from build123d import *

# Parameters (mm, degrees)
EXTRUDE_1_DEPTH     = 20
SKETCH_2_R          = 7
CUT_EXTRUDE_1_DEPTH = 21
SKETCH_3_W          = 30
SKETCH_3_H          = 8
CUT_EXTRUDE_2_DEPTH = 21
FILLET_1_R          = 4
CHAMFER_1_SIZE      = 0.5
M4X0_71_D           = 3.3
M4X0_71_DEPTH       = 13.5
M4X0_71_TIP         = 0.991420021
SKETCH_6_R          = 2
CUT_EXTRUDE_3_DEPTH = 5
SKETCH_7_R          = 2
CUT_EXTRUDE_4_DEPTH = 5
SKETCH_8_R          = 2
EXTRUDE_2_DEPTH     = 5
SKETCH_9_R          = 2
EXTRUDE_3_DEPTH     = 5


with BuildPart() as part:
    # Эскиз1 → Бобышка-Вытянуть1 (new body)
    with BuildSketch(Plane(origin=(0, 0, 0), x_dir=(1, 0, 0), z_dir=(0, 1, 0))):
        with BuildLine():
            Line((0, 0), (14.43375673, -25))
            Line((14.43375673, -25), (65.56624327, -25))
            Line((65.56624327, -25), (80, 0))
            Line((80, 0), (73.07179677, 4))
            Line((73.07179677, 4), (63.396104176, -12.758791171))
            ThreePointArc((63.396104176, -12.758791171), (56.617091212, -7.146468727), (48.291796068, -10))
            Line((48.291796068, -10), (31.708203932, -10))
            ThreePointArc((31.708203932, -10), (23.382908788, -7.146468727), (16.603895824, -12.758791171))
            Line((16.603895824, -12.758791171), (6.92820323, 4))
            Line((6.92820323, 4), (0, 0))
        make_face()
    extrude(amount=EXTRUDE_1_DEPTH)

    # Эскиз2 → Вырез-Вытянуть1 (cut, through all)
    with BuildSketch(Plane(origin=(0, 20, 0), x_dir=(1, 0, 0), z_dir=(0, 1, 0))):
        with Locations((25, -16)):
            Circle(SKETCH_2_R)
        with Locations((55, -16)):
            Circle(SKETCH_2_R)
    extrude(amount=-CUT_EXTRUDE_1_DEPTH, mode=Mode.SUBTRACT)

    # Эскиз3 → Вырез-Вытянуть2 (cut, through all)
    with BuildSketch(Plane(origin=(0, 20, 0), x_dir=(1, 0, 0), z_dir=(0, 1, 0))):
        with Locations((40, -16)):
            Rectangle(SKETCH_3_W, SKETCH_3_H)
    extrude(amount=-CUT_EXTRUDE_2_DEPTH, mode=Mode.SUBTRACT)

    # Скругление1
    fillet_1_edges = [part.edges().sort_by_distance(p)[0] for p in [
        (6.92820323, 10, -4),
        (16.603895824, 10, 12.758791171),
        (31.708203932, 10, 10),
        (48.291796068, 10, 10),
        (63.396104176, 10, 12.758791171),
        (73.07179677, 10, -4),
        (65.56624327, 10, 25),
        (14.43375673, 10, 25),
        (49.255437353, 10, 12),
        (49.255437353, 10, 20),
        (30.744562647, 10, 20),
        (30.744562647, 10, 12),
    ]]
    fillet(fillet_1_edges, radius=FILLET_1_R)

    # Фаска1
    chamfer_1_edges = [part.edges().sort_by_distance(p)[0] for p in [
        (80, 10, 0),
        (0, 10, 0),
    ]]
    chamfer(chamfer_1_edges, length=CHAMFER_1_SIZE)

    # Отверстие обработанное метчиком M4x0.71
    with Locations(Plane(origin=(40, 5, 10), x_dir=(-1, 0, 0), z_dir=(0, 0, -1))):
        with Locations((0, 0), (0, 10)):
            Hole(M4X0_71_D / 2, depth=M4X0_71_DEPTH)
            with Locations((0, 0, -(M4X0_71_DEPTH + M4X0_71_TIP / 2))):  # 118° drill point
                Cone(0, M4X0_71_D / 2, M4X0_71_TIP, mode=Mode.SUBTRACT)

    # Эскиз6 → Вырез-Вытянуть3 (cut)
    with BuildSketch(Plane(origin=(60, 0, 34.641016151), x_dir=(0.5, 0, -0.866025404), z_dir=(0.866025404, 0, 0.5))):
        with Locations((23.441887617, 10)):
            Circle(SKETCH_6_R)
    extrude(amount=-CUT_EXTRUDE_3_DEPTH, mode=Mode.SUBTRACT)

    # Эскиз7 → Вырез-Вытянуть4 (cut)
    with BuildSketch(Plane(origin=(0, 0, 0), x_dir=(0.5, 0, 0.866025404), z_dir=(-0.866025404, 0, 0.5))):
        with Locations((16.558112383, 10)):
            Circle(SKETCH_7_R)
    extrude(amount=-CUT_EXTRUDE_4_DEPTH, mode=Mode.SUBTRACT)

    # Эскиз8 → Бобышка-Вытянуть2 (add)
    with BuildSketch(Plane(origin=(0, 0, 0), x_dir=(0.5, 0, 0.866025404), z_dir=(-0.866025404, 0, 0.5))):
        with Locations((5, 16)):
            Circle(SKETCH_8_R)
    extrude(amount=EXTRUDE_2_DEPTH)

    # Эскиз9 → Бобышка-Вытянуть3 (add)
    with BuildSketch(Plane(origin=(60, 0, 34.641016151), x_dir=(0.5, 0, -0.866025404), z_dir=(0.866025404, 0, 0.5))):
        with Locations((35, 16)):
            Circle(SKETCH_9_R)
    extrude(amount=EXTRUDE_3_DEPTH)


solid = part.part
Verification items for the finished model (mm, model axes). A direction names the side the tool comes from. Give positions to 0.01 mm unless a question says otherwise; leave off trailing zeros. Order: outer loops, then holes, each group sorted by start corner. A loop starts at its lowest first (then second) coordinate and runs counter-clockwise, first axis right, second up. Notation, with made-up numbers: M -5,61.25 L 46,61.25 A17 cw 46,89.25 Z; hole C 40,76.5 d5. An arc over 180 degrees is marked long. Answer as a JSON object with one key per item and string values. Group by question number.
1) Cross-section at A-A (x = 55). Enter the section's corners in (y, z).
2) Cross-section at B-B (x = 26.5). Enter the section's corners in (y, z).
3) Access from +Z, -Z, +X, -X, +Y, -Y to the whole of each face (thin tool, end or side, straight path). Record for faces 4 (the face through (40, 10, 25)), 5 (the face through (38.35, 5.07, 21.77)), 6 (the face through (67.38, 10.03, 11.86)), 7 (the face through (62, 10, 16)), 8 (the face through (40, 10, 10)).
4) Depth check by flat-ended pin: pin 1 Ø6 at (x, y) = (73, 11.5) entering from +Z; pin 2 Ø3 at (y, z) = (17.5, 6.5) entering from +X; pin 3 Ø2.5 at (x, y) = (40, 5) entering from -Z; pin 4 Ø8.5 at (x, z) = (55, 16) entering from +Y. Enter the tip coordinate at first touch or a pass-through.
5) Scan lines: line 1 along Y through (x, z) = (40, 10.6); line 2 along Z through (x, y) = (54.5, 3.5); line 3 along X through (y, z) = (17.75, 7.75). Record each from-to range of solid material in increasing order. Write a range as [from, to].
6) Mould release check, pull along Z, two halves, no side actions. Record for faces 1 (the face through (65.28, 10.14, 24.45)), 2 (the face through (31.092, 10.14, 20.275)), 3 (the face through (31.93, 10.14, 9.756)): released by +Z, released by -Z, zero draft, split by the parting line, or undercut.
Result sheet:
{
 "1": {"outline": "M 0,7 L 20,7 L 20,9 L 0,9 Z; M 0,23 L 20,23 L 20,25 L 0,25 Z"},
 "2": {"outline": "M 0,7.13 L 20,7.13 L 20,9.16 L 0,9.16 Z; M 0,22.84 L 20,22.84 L 20,25 L 0,25 Z"},
 "3": {"face 4": "+Z, +X, -X, +Y, -Y", "face 5": "-Z", "face 6": "none", "face 7": "+Y, -Y", "face 8": "-Z, +Y, -Y"},
 "4": {"pin 1": "stops at z = 17.32", "pin 2": "stops at x = 82.76", "pin 3": "stops at z = 23.74", "pin 4": "passes through"},
 "5": {"line 1": "y = [0, 3.35], [6.65, 13.35], [16.65, 20]", "line 2": "z = [7.01, 9.02], [22.98, 25]", "line 3": "x = [4.47, 13.71], [21.4, 28.6], [51.4, 58.6], [66.29, 75.53]"},
 "6": {"face 1": "released by +Z", "face 2": "undercut", "face 3": "released by -Z"}
}
